Autodesk Fusion 360 part; units mm, degrees
sketch "Sketch1" plane through (0, 0, 0) normal (0, 1, 0) x (1, 0, 0)
  line L0 (-70, -50) -> (-12, -50)
  line L1 (-12, -50) -> (-12, -1)
  line L2 (-12, -1) -> (-70, -1)
  line L3 (-70, -1) -> (-70, -50)
  circle A0 centre (-70, -50) radius 1.35
  circle A1 centre (-12, -50) radius 1.35
  circle A2 centre (-70, -1) radius 1.35
  circle A3 centre (-12, -1) radius 1.35
  line L4 (-41, -50) -> (-41, -25.5)
  line L5 (0, -53) -> (-82, -53)
  line L6 (-82, -53) -> (-82, 2)
  line L7 (-82, 2) -> (0, 2)
  line L8 (0, 2) -> (0, -53)
  line L9 (0, -53) -> (-82, 2) construction
  line L10 (-82, -53) -> (0, 2) construction
  circle A4 centre (-77.6409, -25.5) radius 2
  circle A5 centre (-4.3591, -25.5) radius 2
  point P0 (-41, -25.5)
  dimension "d1" = 58
  dimension "d2" = 49
  dimension "d3" = 2.7
  dimension "d4" = 2.7
  dimension "d5" = 2.7
  dimension "d6" = 2.7
  dimension "d7" = 4
extrude "Extrude1" add sketch "Sketch1" along normal blind 2 contours L0 L1 L2 L3 A0 A1 A2 A3 | L5 L6 L7 L8
sketch "Sketch2" plane through (0, 0, 0) normal (0, -1, 0) x (1, 0, 0)
  circle A0 centre (-4.3591, 25.5) radius 2
  circle A1 centre (-70, 50) radius 1.35
  circle A2 centre (-77.6409, 25.5) radius 2
  circle A3 centre (-12, 50) radius 1.35
  circle A4 centre (-70, 1) radius 1.35
  circle A5 centre (-12, 1) radius 1.35
  line L0 (-82, -2) -> (0, -2)
  line L1 (0, -2) -> (0, 53)
  line L2 (0, 53) -> (-82, 53)
  line L3 (-82, 53) -> (-82, -2)
  circle A6 centre (-12, 50) radius 3
  circle A7 centre (-12, 50) radius 1.35
  circle A8 centre (-12, 1) radius 1.35
  circle A9 centre (-12, 1) radius 2
  circle A10 centre (-70, 1) radius 1.35
  circle A11 centre (-70, 1) radius 2
  circle A12 centre (-70, 50) radius 1.35
  circle A13 centre (-70, 50) radius 2
  circle A14 centre (-12, 50) radius 2
  dimension "d10" = 4
  dimension "d11" = 4
  dimension "d12" = 4
extrude "Extrude2" add sketch "Sketch2" along normal blind 3 contours A9 | A11 | A13 | A14
extrude "Extrude3" add 1 faces at (0, 0.6667, 16.3333) along direction (1, 0, 0) blind 6
extrude "Extrude4" add 1 faces at (-82, 0.6667, 34.6667) along direction (-1, 0, 0) blind 6
extrude "Extrude5" add 1 faces at (-25.3333, 0.6667, -2) along direction (0, 0, -1) blind 5
extrude "Extrude6" add 1 faces at (-25.3333, 0.6667, 53) along direction (0, 0, 1) blind 5
sketch "Sketch3" plane through (0, 0, 0) normal (0, -1, 0) x (1, 0, 0)
  circle A0 centre (-12, 1) radius 2
  circle A1 centre (-12, 50) radius 2
  circle A2 centre (-70, 1) radius 2
  circle A3 centre (-70, 50) radius 2
  circle A4 centre (-4.3591, 25.5) radius 2
  circle A5 centre (-77.6409, 25.5) radius 2
  line L0 (6, -7) -> (6, 58)
  line L1 (6, 58) -> (-88, 58)
  line L2 (-88, 58) -> (-88, -7)
  line L3 (-88, -7) -> (6, -7)
  circle A6 centre (-85, 55) radius 2
  line L4 (-41, 58) -> (-41, 35)
  line L5 (-88, 25.5) -> (-67.9088, 25.5)
  circle A7 centre (3, 55) radius 2
  circle A8 centre (-85, -4) radius 2
  circle A9 centre (3, -4) radius 2
extrude "Extrude7" cut sketch "Sketch3" against normal blind 15 contours A6 | A7 | A8 | A9
Source: CAD feature listing. Evaluate the final solid. Frame: model axes, mm. A direction names the side the tool comes from. Give positions to 0.01 mm unless a question says otherwise; leave off trailing zeros. Write each loop counter-clockwise with the first axis right and the second up, starting at its lowest first coordinate (ties: lowest second). Pieces come first, ordered by that corner, then holes. Notation, with made-up numbers: M -24,58.25 L 18,58.25 A14 cw 18,74.25 Z; hole C 39.5,-38 d3. An arc over 180 degrees is marked long. Return JSON: item names as keys, results as strings. Group by question number.
1) Cut plane D-D, the plane z = -4. Output: boundary loops of the cut face in (x, y).
2) Cut plane C-C, the plane x = -12. Output: boundary loops of the cut face in (y, z), plus the area to 3 significant figures.
3) Cut plane A-A, the plane y = -1.8. Output: boundary loops of the cut face in (x, z), plus the area to 3 significant figures.
4) Pull-direction query (X, two-part tool) for faces 3 (the face through (-40, 2, 25)), 4 (the face through (-68.753, -0.535, 0.483)), 5 (the face through (6, 1, 25)); classes: pulls with the +X half, pulls with the -X half, needs draft (parallel to the pull), parting line crosses it, or undercut.
5) Set-up query: faces 1 (the face through (1.4, 1, -5.2)), 2 (the face through (-68.092, -1.479, 0.399)). Return all of +Z, -Z, +X, -X, +Y, -Y with unobstructed straight access to the full face (end or side cutting, diameter ignored); none if empty.
6) Pin query (flat end, axial travel): P1, Ø5, axis at x = -77.64, z = 25.5, coming from the -Y side; P2, Ø1.6, axis at x = -70, z = 1, coming from the -Y side. Return the tip coordinate at first contact, or that it passes through.
7) Material intervals for line 1 along Z through (x, y) = (-70, -0.35); line 2 along Z through (x, y) = (-85, 1.35); line 3 along X through (y, z) = (-1.05, 1.5), sorted ascending. Write a range as [from, to].
8) Cut plane B-B, the plane z = 50. Output: boundary loops of the cut face in (x, y).
Recorded:
{
 "1": {"outline": "M -88,0 L -87,0 L -87,2 L -88,2 Z; M -83,0 L 1,0 L 1,2 L -83,2 Z; M 5,0 L 6,0 L 6,2 L 5,2 Z"},
 "2": {"outline": "M -3,-1 L 0,-1 L 0,-7 L 2,-7 L 2,-0.35 L -3,-0.35 Z; M -3,2.35 L 2,2.35 L 2,48.65 L -3,48.65 L -3,48 L 0,48 L 0,3 L -3,3 Z; M -3,51.35 L 2,51.35 L 2,58 L 0,58 L 0,52 L -3,52 Z", "area": "127 mm²"},
 "3": {"outline": "C -70,1 d4; C -70,50 d4; C -12,1 d4; C -12,50 d4; hole C -70,1 d2.7; hole C -70,50 d2.7; hole C -12,1 d2.7; hole C -12,50 d2.7", "area": "27.4 mm²"},
 "4": {"face 3": "needs draft", "face 4": "undercut", "face 5": "pulls with the +X half"},
 "5": {"face 1": "+Y, -Y", "face 2": "-Y"},
 "6": {"P1": "stops at y = 0", "P2": "passes through"},
 "7": {"line 1": "z = [-1, -0.35], [2.35, 3], [48, 48.65], [51.35, 52]", "line 2": "z = [-7, -6], [-2, 53], [57, 58]", "line 3": "x = [-71.94, -71.25], [-68.75, -68.06], [-13.94, -13.25], [-10.75, -10.06]"},
 "8": {"outline": "M -88,0 L -72,0 L -72,-3 L -71.35,-3 L -71.35,2 L -88,2 Z; M -68.65,-3 L -68,-3 L -68,0 L -14,0 L -14,-3 L -13.35,-3 L -13.35,2 L -68.65,2 Z; M -10.65,-3 L -10,-3 L -10,0 L 6,0 L 6,2 L -10.65,2 Z"}
}
